```python
from build123d import *

# Parameters (mm, degrees)
EXTRUDE_1_DEPTH        = 800
SKETCH_2_R             = 3
CUT_EXTRUDE_1_DEPTH    = 3
CUT_EXTRUDE_2_REACH    = 802.049
SKETCH_3_R             = 1.6
PATTERN_LINEAR_1_COUNT = 32
PATTERN_LINEAR_1_PITCH = 25
SKETCH_5_W             = 302.225759888
SKETCH_5_H             = 503.019586662
CUT_EXTRUDE_3_DEPTH    = 10
SKETCH_6_W             = 27.58058317
SKETCH_6_H             = 207.193316332
CUT_EXTRUDE_4_DEPTH    = 10


with BuildPart() as part:
    # 草图1 → 凸台-拉伸1 (new body)
    with BuildSketch(Plane.XY):
        Polygon((-6.5, 4.5), (6.5, 4.5), (6.5, 1.2), (2.5, 1.2), (2.5, -2.076527235), (6.5, -3), (6.5, -4.5), (-6.5, -4.5), (-6.5, -3), (-2.5, -2.076527235), (-2.5, 1.2), (-6.5, 1.2), align=None)
    extrude(amount=EXTRUDE_1_DEPTH)

    # 草图2 → 切除-拉伸1 (cut)
    with BuildSketch(Plane(origin=(0, 4.5, 0), x_dir=(1, 0, 0), z_dir=(0, 1, 0))):
        with Locations(Location((0, -790, 0), (0, 0, 270))):
            Circle(SKETCH_2_R)
    cut_extrude_1 = extrude(amount=-CUT_EXTRUDE_1_DEPTH, mode=Mode.SUBTRACT)

    # 草图3 → 切除-拉伸2 (cut, up to next)
    with BuildSketch(Plane(origin=(0, 1.5, 0), x_dir=(1, 0, 0), z_dir=(0, 1, 0)), mode=Mode.PRIVATE) as cut_extrude_2_sk1:
        with Locations(Location((0, -790, 0), (0, 0, 270))):
            Circle(SKETCH_3_R)
    cut_extrude_2_tool1 = extrude(cut_extrude_2_sk1.sketch, amount=-CUT_EXTRUDE_2_REACH, mode=Mode.PRIVATE) & part.part
    cut_extrude_2 = cut_extrude_2_tool1.solids().sort_by_distance((0, 1.5, 790))[0]
    add(cut_extrude_2, mode=Mode.SUBTRACT)

    # 阵列(线性)1: 切除-拉伸1, 切除-拉伸2 ×32
    with Locations(*[(0, 0, -i * PATTERN_LINEAR_1_PITCH) for i in range(1, PATTERN_LINEAR_1_COUNT)]):
        add(cut_extrude_1, mode=Mode.SUBTRACT)
        add(cut_extrude_2, mode=Mode.SUBTRACT)

    # 草图5 → 切除-拉伸3 (cut)
    with BuildSketch(Plane(origin=(0, 4.5, 0), x_dir=(1, 0, 0), z_dir=(0, 1, 0))):
        with Locations((0, -941.509793331)):
            Rectangle(SKETCH_5_W, SKETCH_5_H)
    extrude(amount=-CUT_EXTRUDE_3_DEPTH, mode=Mode.SUBTRACT)

    # 草图6 → 切除-拉伸4 (cut)
    with BuildSketch(Plane(origin=(0, 4.5, 0), x_dir=(1, 0, 0), z_dir=(0, 1, 0))):
        with Locations((0, -51.403341834)):
            Rectangle(SKETCH_6_W, SKETCH_6_H)
    extrude(amount=-CUT_EXTRUDE_4_DEPTH, mode=Mode.SUBTRACT)


solid = part.part
```
The model under review builds one solid part; all positions refer to its coordinate system, in mm. Give positions to 0.01 mm unless a question says otherwise; leave off trailing zeros. Write each loop counter-clockwise with the first axis right and the second up, starting at its lowest first coordinate (ties: lowest second). Pieces come first, ordered by that corner, then holes. Notation, with made-up numbers: (-30, 74) - (21, 74) arc R36 ccw to (21, 110) - close; hole circle Ø4 at (49.25, 62.25). An arc over 180 degrees is marked (long way). Answer in a Markdown table with one row per item. Add a question column.
1. We need section A-A on z = 381.5. Write out the cut boundary in (x, y), then the cut area to 3 significant figures.
2. Wall thickness on line 1 along Y through (x, z) = (-4.5, 396.5); line 2 along X through (y, z) = (0, 290); line 3 along X through (y, z) = (3.4, 365): over which ranges is each line inside the solid? List them lowest first. Write a range as [from, to].
3. Insertion check: P1, Ø1, axis at y = -0.5, z = 292, coming from the -X side; P2, Ø4, axis at x = 3, y = -1, coming from the +Z side; P3, Ø3.5, axis at x = 0, z = 365, coming from the +Y side. Each pin has a flat end and moves straight along its axis. Give the tip position at first contact, or say it passes through.
Ans:
| question | item | result |
|---|---|---|
| 1 | outline | (-6.5, -4.5) - (6.5, -4.5) - (6.5, -3) - (2.5, -2.08) - (2.5, 1.2) - (6.5, 1.2) - (6.5, 4.5) - (-6.5, 4.5) - (-6.5, 1.2) - (-2.5, 1.2) - (-2.5, -2.08) - (-6.5, -3) - close |
| 1 | area | 87.1 mm^2 |
| 2 | line 1 | y = [-4.5, -2.54], [1.2, 4.5] |
| 2 | line 2 | x = [-2.5, -1.6], [1.6, 2.5] |
| 2 | line 3 | x = [-6.5, -3], [3, 6.5] |
| 3 | P1 | stops at x = -2.5 |
| 3 | P2 | stops at z = 690 |
| 3 | P3 | stops at y = 1.5 |
